CAD build for the part. Positions are in the model's coordinates, mm. A direction names the side the tool comes from. Coordinates: 2 decimals unless noted, no trailing zeros. Order: outer loops, then holes, each group sorted by start corner. A loop starts at its lowest first (then second) coordinate and runs counter-clockwise, first axis right, second up. Notation, with made-up numbers: (30, 18) -> (77, 18) arc R26 cw to (77, 50) -> close; hole circle Ø8 at (-27.75, 37.25). An arc over 180 degrees is marked (long way). Use one line per item in the form item = value. Start each with the question number.
from build123d import *

# Parameters (mm, degrees)
SKETCH7_W           = 100
SKETCH7_H           = 100
BOSS_EXTRUDE1_DEPTH = 100
SKETCH8_R           = 15
CUT_EXTRUDE1_DEPTH  = 10
SKETCH9_R           = 10
CUT_EXTRUDE2_DEPTH  = 10
SKETCH10_R          = 10
CUT_EXTRUDE3_DEPTH  = 10
SKETCH13_R          = 12.5
CUT_EXTRUDE4_DEPTH  = 10
SKETCH14_R          = 12.5
CUT_EXTRUDE5_DEPTH  = 10
SKETCH16_R          = 12.5
CUT_EXTRUDE11_DEPTH = 10


with BuildPart() as part:
    # Sketch7 → Boss-Extrude1 (new body)
    with BuildSketch(Plane(origin=(0, 0, 0), x_dir=(1, 0, 0), z_dir=(0, 1, 0))):
        Rectangle(SKETCH7_W, SKETCH7_H)
    extrude(amount=BOSS_EXTRUDE1_DEPTH)

    # Sketch8 → Cut-Extrude1 (cut)
    with BuildSketch(Plane(origin=(0, 100, 0), x_dir=(1, 0, 0), z_dir=(0, 1, 0))):
        with Locations(Location((0, 0, 0), (0, 0, 270))):
            Circle(SKETCH8_R)
    extrude(amount=-CUT_EXTRUDE1_DEPTH, mode=Mode.SUBTRACT)

    # Sketch9 → Cut-Extrude2 (cut)
    with BuildSketch(Plane(origin=(50, 0, 0), x_dir=(0, 0, -1), z_dir=(1, 0, 0))):
        with Locations((0, 50)):
            Circle(SKETCH9_R)
        with Locations((24.748737342, 74.748737342)):
            Circle(SKETCH9_R)
        with Locations((-24.748737342, 25.251262658)):
            Circle(SKETCH9_R)
    extrude(amount=-CUT_EXTRUDE2_DEPTH, mode=Mode.SUBTRACT)

    # Sketch10 → Cut-Extrude3 (cut)
    with BuildSketch(Plane.XY.offset(50)):
        with Locations((-25.023456699, 24.976543301)):
            Circle(SKETCH10_R)
        with Locations((24.474017984, 74.474017984)):
            Circle(SKETCH10_R)
    extrude(amount=-CUT_EXTRUDE3_DEPTH, mode=Mode.SUBTRACT)

    # Sketch13 → Cut-Extrude4 (cut)
    with BuildSketch(Plane(origin=(0, 0, 0), x_dir=(-1, 0, 0), z_dir=(0, -1, 0))):
        with Locations(Location((25, -25, 0), (0, 0, 90))):
            Circle(SKETCH13_R)
        with Locations(Location((-25, -25, 0), (0, 0, 90))):
            Circle(SKETCH13_R)
        with Locations(Location((25, 25, 0), (0, 0, 90))):
            Circle(SKETCH13_R)
        with Locations(Location((-25, 25, 0), (0, 0, 90))):
            Circle(SKETCH13_R)
    extrude(amount=-CUT_EXTRUDE4_DEPTH, mode=Mode.SUBTRACT)

    # Sketch14 → Cut-Extrude5 (cut)
    with BuildSketch(Plane(origin=(0, 0, -50), x_dir=(-1, 0, 0), z_dir=(0, 0, -1))):
        with Locations((25, 25)):
            Circle(SKETCH14_R)
        with Locations((-25, 25)):
            Circle(SKETCH14_R)
        with Locations((25, 75)):
            Circle(SKETCH14_R)
        with Locations((-25, 75)):
            Circle(SKETCH14_R)
        with Locations((0, 50)):
            Circle(SKETCH14_R)
    extrude(amount=-CUT_EXTRUDE5_DEPTH, mode=Mode.SUBTRACT)

    # Sketch16 → Cut-Extrude11 (cut)
    with BuildSketch(Plane.ZY.offset(50)):
        with Locations((-35, 75)):
            Circle(SKETCH16_R)
        with Locations((0, 75)):
            Circle(SKETCH16_R)
        with Locations((35, 75)):
            Circle(SKETCH16_R)
        with Locations((-35, 25)):
            Circle(SKETCH16_R)
        with Locations((0, 25)):
            Circle(SKETCH16_R)
        with Locations((35, 25)):
            Circle(SKETCH16_R)
    extrude(amount=-CUT_EXTRUDE11_DEPTH, mode=Mode.SUBTRACT)


solid = part.part
1) Probe L1, parallel to Y at x = -45.25, z = 35; L2, parallel to Y at x = 46, z = 0; L3, parallel to Y at x = 17, z = -19. List the from-to ranges inside material, lowest first.
2) Cut at D-D on x = -25. Give the cut face in (y, z).
3) 3-axis set-ups, long thin cutter, end or side, ignore diameter. For faces 4 (the face through (40, 75, -25)), 5 (the face through (-45.07, 87.394, -1.627)), 6 (the face through (-23.373, 87.394, -45.07)), 7 (the face through (0.66, 95.07, -14.985)), 8 (the face through (17.394, 4.93, -15.08)): which of +Z, -Z, +X, -X, +Y, -Y reach the whole face in a straight line?
4) Drop flat-ended pins along their axis: P1, Ø20, axis at x = 25, z = 25, coming from the -Y side; P2, Ø6, axis at y = 21.5, z = 24.5, coming from the +X side; P3, Ø12.5, axis at y = 70.5, z = -36.5, coming from the -X side. Give the stop position or say it passes through.
5) Cut at B-B on x = -7. Give the cut face in (y, z).
6) Cut at A-A on z = 0. Give the cut face in (x, y).
7) Two-plate mould, pull along Y, no slides. Class faces 1 (the face through (-1, 0, -1)), 2 (the face through (12.797, 4.93, 27.71)), 3 (the face through (-25, 25, 40)): released by +Y, released by -Y, zero draft, split by the parting line, or undercut.
Values follow:
q1.L1 = 0 to 12.5, 37.5 to 62.5, 87.5 to 100
q1.L2 = 0 to 40, 60 to 100
q1.L3 = 10 to 100
q2.outline = (0, -50) -> (12.5, -50) -> (12.5, -40) -> (37.5, -40) -> (37.5, -50) -> (62.5, -50) -> (62.5, -40) -> (87.5, -40) -> (87.5, -50) -> (100, -50) -> (100, 50) -> (34.98, 50) -> (34.98, 40) -> (14.98, 40) -> (14.98, 50) -> (0, 50) -> (0, 37.5) -> (10, 37.5) -> (10, 12.5) -> (0, 12.5) -> (0, -12.5) -> (10, -12.5) -> (10, -37.5) -> (0, -37.5) -> close
q3.face_4 = +X
q3.face_5 = -X
q3.face_6 = -Z
q3.face_7 = +Y
q3.face_8 = -Y
q4.P1 = 10
q4.P2 = 40
q4.P3 = -40
q5.outline = (0, -50) -> (39.64, -50) -> (39.64, -40) -> (60.36, -40) -> (60.36, -50) -> (100, -50) -> (100, -13.27) -> (90, -13.27) -> (90, 13.27) -> (100, 13.27) -> (100, 50) -> (0, 50) -> close
q6.outline = (-50, 0) -> (50, 0) -> (50, 40) -> (40, 40) -> (40, 60) -> (50, 60) -> (50, 100) -> (15, 100) -> (15, 90) -> (-15, 90) -> (-15, 100) -> (-50, 100) -> (-50, 87.5) -> (-40, 87.5) -> (-40, 62.5) -> (-50, 62.5) -> (-50, 37.5) -> (-40, 37.5) -> (-40, 12.5) -> (-50, 12.5) -> close
q7.face_1 = released by -Y
q7.face_2 = zero draft
q7.face_3 = undercut
